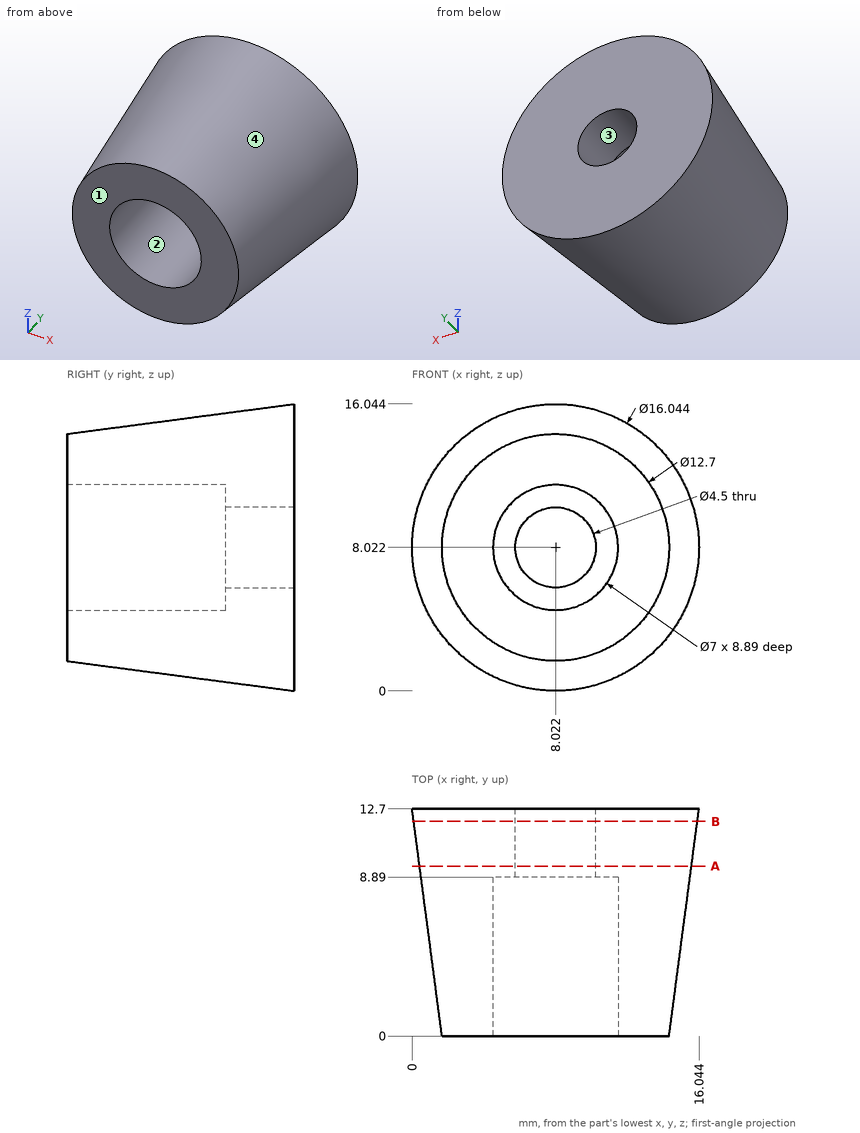
Part print with two shaded views. Sizes in mm from the minimum x, y, z corner. Coordinates: 2 decimals unless noted, no trailing zeros. Write each loop counter-clockwise with the first axis right and the second up, starting at its lowest first coordinate (ties: lowest second). Pieces come first, ordered by that corner, then holes. Notation, with made-up numbers: (70, 8.5) - (76, 8.5) arc R16 ccw to (76, 24.5) - close; hole circle Ø10 at (82, 18.5). An arc over 180 degrees is marked (long way). Put each result on its own line as item: value.
1. Two-plate mould, pull along X, no slides. Class the marked faces 1, 2, 3 and 4: +X half, -X half, draft (parallel to the pull), parting line (faces both ways), or undercut.
Final values:
face 1: draft
face 2: undercut
face 3: undercut
face 4: parting line
2. Probe line 1 along X through (y, z) = (8.5, 9.5); line 2 along Z through (x, y) = (5.5, 1.75) (3 decimals); line 3 along X through (y, z) = (2.75, 11). List the from-to ranges inside material, lowest first. Write a range as [from, to].
Final values:
line 1: x = [0.7, 4.85], [11.19, 15.34]
line 2: z = [1.944, 5.595], [10.449, 14.1]
line 3: x = [2.01, 6.18], [9.86, 14.04]
3. Flat gauge pins, fed straight in: pin 1 Ø2 at (x, z) = (9, 7) entering from -Y; pin 2 Ø6 at (x, z) = (8.02, 8.02) entering from +Y; pin 3 Ø5 at (y, z) = (10, 13) entering from -X; pin 4 Ø4 at (x, y) = (13.5, 8.5) entering from +Z. Where does each tip first touch, or does it go through?
Final values:
pin 1: stops at y = 8.89
pin 2: stops at y = 12.7
pin 3: stops at x = 0.7
pin 4: stops at z = 14.67
4. Band-saw the part on B-B (y = 12). Write the cut outline in (x, z).
Final values:
outline: circle Ø15.86 at (8.02, 8.02); hole circle Ø4.5 at (8.02, 8.02)
5. Band-saw the part on A-A (y = 9.5). Write the cut outline in (x, z).
Final values:
outline: circle Ø15.2 at (8.02, 8.02); hole circle Ø4.5 at (8.02, 8.02)
